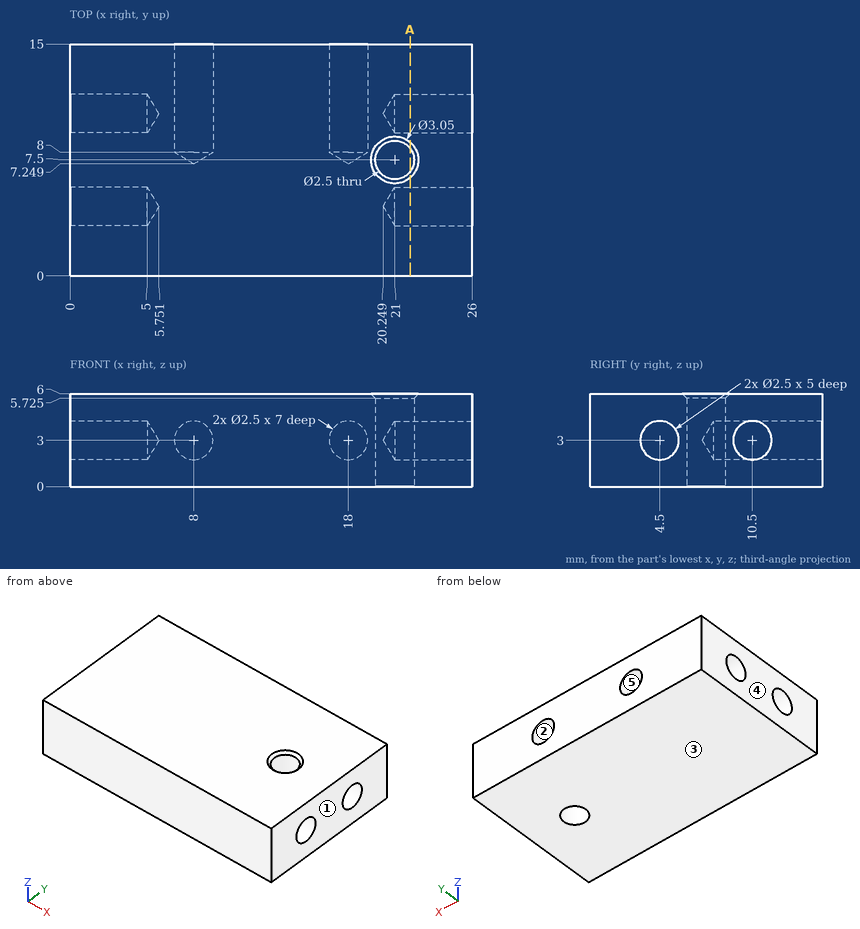
Drawing for the job (mm, zero at the part's lowest x, y, z). A direction names the side the tool comes from. Give positions to 0.01 mm unless a question says otherwise; leave off trailing zeros. Use one line per item in the form item = value.
Item 1: Probe probe 1 along Y at (x, z) = (1.25, 3); probe 2 along X at (y, z) = (7.5, 3.65); probe 3 along X at (y, z) = (10, 1.95). List the from-to ranges inside material, lowest first. Write a range as from..to.
Solution:
probe_1 = 0..3.25, 5.75..9.25, 11.75..15
probe_2 = 0..19.75, 22.25..26
probe_3 = 5.05..7.32, 8.68..17.32, 18.68..20.95
Item 2: Two-plate mould, pull along Z, no slides. Class the marked faces 1, 2 and 3: released by +Z, released by -Z, zero draft, split by the parting line, or undercut.
Solution:
face_1 = zero draft
face_2 = undercut
face_3 = released by -Z
Item 3: Slice it at A-A on x = 22. Count the separate pieces of the cut face and the enclosed holes in it, and give its area (3 significant figures).
Solution:
separate_pieces = 2
enclosed_holes = 2
area = 71.1 mm2
Item 4: Which spindle directions (+Z, -Z, +X, -X, +Y, -Y) get a long thin tool onto all of the face, cutting with end or side? Do the marked faces 4 and 5. Say none if no direction does.
Solution:
face_4 = +Z, -Z, -X, +Y, -Y
face_5 = +Y
Item 5: Pin check, flat tips, straight feed: pin 1 Ø1.5 at (x, z) = (18, 3) entering from +Y; pin 2 Ø2 at (x, z) = (8, 3) entering from +Y; pin 3 Ø2 at (y, z) = (10.5, 3) entering from -X; pin 4 Ø1.5 at (x, y) = (21, 7.5) entering from +Z. Stop position of each tip, or through.
Solution:
pin_1 = 7.7
pin_2 = 7.85
pin_3 = 5.15
pin_4 = through
